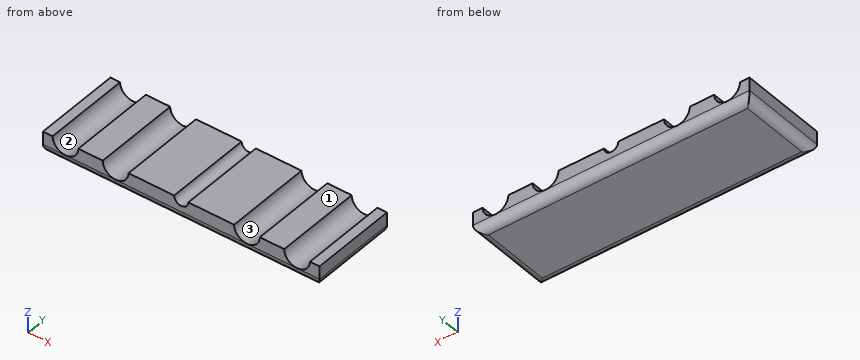
from build123d import *

# Parameters (mm, degrees)
ESQUISSE1_W             = 160
ESQUISSE1_H             = 50
BOSS_EXTRU_1_DEPTH      = 12.5
ESQUISSE2_R             = 7.45
ESQUISSE2_R_2           = 4.1
ENL_V_MAT_EXTRU_1_DEPTH = 169.09595474
CONG_1_R                = 5


with BuildPart() as part:
    # Esquisse1 → Boss.-Extru.1 (new body)
    with BuildSketch(Plane.XY):
        with Locations((-80, -25)):
            Rectangle(ESQUISSE1_W, ESQUISSE1_H)
    extrude(amount=BOSS_EXTRU_1_DEPTH)

    # Esquisse2 → Enlèv. mat.-Extru.1 (cut, through all)
    with BuildSketch(Plane(origin=(0, 0, 0), x_dir=(1, 0, 0), z_dir=(0, 1, 0))):
        with Locations((-147, -12.5)):
            Circle(ESQUISSE2_R)
        with Locations((-118, -12.5)):
            Circle(ESQUISSE2_R)
        with Locations((-13, -12.5)):
            Circle(ESQUISSE2_R)
        with Locations((-42, -12.5)):
            Circle(ESQUISSE2_R)
        with Locations((-80, -12.5)):
            Circle(ESQUISSE2_R_2)
    extrude(amount=-ENL_V_MAT_EXTRU_1_DEPTH, mode=Mode.SUBTRACT)

    # Congé1
    cong_1_edges = [part.edges().sort_by_distance(p)[0] for p in [
        (-80, -50, 0),
        (-160, -25, 0),
        (-80, 0, 0),
        (0, -25, 0),
    ]]
    fillet(cong_1_edges, radius=CONG_1_R)


solid = part.part
For this review, take the finished solid that the model builds, in its own axes (mm). Face numbers are marked on the shaded views. Coordinates: 2 decimals unless noted, no trailing zeros. Order: outer loops, then holes, each group sorted by start corner. A loop starts at its lowest first (then second) coordinate and runs counter-clockwise, first axis right, second up. Notation, with made-up numbers: (-31.75, -14.75) - (-24.75, -14.75) arc R21 ccw to (-24.75, 0.25) - close; hole circle Ø7 at (57, 55). An arc over 180 degrees is marked (long way). Answer as CSV lines item,"result". Start each with the question number.
1) Draft analysis for pull direction X (two halves, no side actions). For the marked faces 1, 2 and 3, state which applies: +X half, -X half, draft (parallel to the pull), parting line (faces both ways), or undercut.
2) To check wall thickness, follow line 1 along X through (y, z) = (-23.5, 12); line 2 along X through (y, z) = (-37, 7.5); line 3 along X through (y, z) = (-37, 11). State the ranges of each line that lie inside material, in increasing order. Write a range as [from, to].
3) Add section A-A (x = -105.5). State the section outline as (y, z) points, then the cut area to 3 significant figures.
4) Add section C-C (x = -42). State the section outline as (y, z) points.
5) Add section B-B (y = -32). State the section outline as (x, z) points, then the cut area to 3 significant figures.
6) Insertion check: P1, Ø2, axis at y = -37, z = 2.5, coming from the +X side. The pin has a flat end and moves straight along its axis. Give the tip position at first contact, or say it passes through.
Result:
1,face 1,"draft"
1,face 2,"undercut"
1,face 3,"undercut"
2,line 1,"[-160, -154.43], [-139.57, -125.43], [-110.57, -84.07], [-75.93, -49.43], [-34.57, -20.43], [-5.57, 0]"
2,line 2,"[-160, -152.52], [-141.48, -123.52], [-112.48, -47.52], [-36.48, -18.52], [-7.48, 0]"
2,line 3,"[-160, -154.3], [-139.7, -125.3], [-110.7, -83.82], [-76.18, -49.3], [-34.7, -20.3], [-5.7, 0]"
3,outline,"(-50, 5) arc R5 ccw to (-45, 0) - (-5, 0) arc R5 ccw to (0, 5) - (0, 12.5) - (-50, 12.5) - close"
3,area,"614 mm^2"
4,outline,"(-50, 5) arc R5 ccw to (-45, 0) - (-5, 0) arc R5 ccw to (0, 5) - (0, 5.05) - (-50, 5.05) - close"
5,outline,"(-160, 5) arc R5 ccw to (-155, 0) - (-5, 0) arc R5 ccw to (0, 5) - (0, 12.5) - (-5.55, 12.5) arc R7.45 cw to (-20.45, 12.5) - (-34.55, 12.5) arc R7.45 cw to (-49.45, 12.5) - (-75.9, 12.5) arc R4.1 cw to (-84.1, 12.5) - (-110.55, 12.5) arc R7.45 cw to (-125.45, 12.5) - (-139.55, 12.5) arc R7.45 cw to (-154.45, 12.5) - (-160, 12.5) - close"
5,area,"1,610 mm^2"
6,P1,"x = -0.23"
